from build123d import *

# Parameters (mm, degrees)
CORTE_EXTRUS_O1_DEPTH      = 14.238697312
CORTE_EXTRUS_O1_DEPTH_BACK = 14.238697312
ESBO_O2_W                  = 3.17038165
ESBO_O2_H                  = 1.5


with BuildPart() as part:
    # Esboço1 → Revolução1 (revolve)
    with BuildSketch(Plane.XY):
        with BuildLine():
            Line((0, 0), (0, 2.5))
            Line((0, 2.5), (8, 2.5))
            Line((8, 2.5), (8, 3.953675657))
            ThreePointArc((8, 3.953675657), (10.812174165, 2.798528059), (12, 0))
            Line((12, 0), (0, 0))
        make_face()
    revolve(axis=Axis((12, 0, 0), (-1, 0, 0)))

    # Esboço2 → Corte-extrusão1 (cut, two sides: drawn at the far end of the back side and taken through both)
    with BuildSketch(Plane.XY.offset(-CORTE_EXTRUS_O1_DEPTH_BACK)):
        with Locations((11.06193306, 0)):
            Rectangle(ESBO_O2_W, ESBO_O2_H)
    extrude(amount=CORTE_EXTRUS_O1_DEPTH + CORTE_EXTRUS_O1_DEPTH_BACK, mode=Mode.SUBTRACT)


solid = part.part
Work out the finished part from the listing and answer in its coordinate system (mm). A direction names the side the tool comes from. Coordinates: 2 decimals unless noted, no trailing zeros. Write each loop counter-clockwise with the first axis right and the second up, starting at its lowest first coordinate (ties: lowest second). Pieces come first, ordered by that corner, then holes. Notation, with made-up numbers: M 14,13 L 45,13 A37 cw 45,52 Z; hole C 7.25,25 d2. An arc over 180 degrees is marked long. Use one line per item in the form item = value. Start each with the question number.
1. Straight lines are drawn through the part: probe 1 along Y at (x, z) = (10, 2.25); probe 2 along X at (y, z) = (0.5, 1); probe 3 along Y at (x, z) = (10, 0.25). For each, find the intervals that lie inside material, in ascending order. Write a range as from..to.
2. The mould has two halves that part along Y. Classify faces 1 (the face through (4.06, -0.54, 2.44)), 2 (the face through (10, 0.75, 0)), 3 (the face through (0, 0, 0)), 4 (the face through (9.477, 0, 0)): released by +Y, released by -Y, zero draft, split by the parting line, or undercut.
3. A tool of negligible diameter and unlimited length cuts with its end or side. For faces 5 (the face through (8, 0, 3)), 6 (the face through (10, -0.75, 0)), from which of +Z, -Z, +X, -X, +Y, -Y can it reach the whole face along a straight path? Write none if from no direction.
4. The part is cut by section A-A (x = 4). Give the vertices of the cut face in (y, z).
5. Each of these flat-tipped pins is pushed along its axis until it touches: P1, Ø1, axis at y = 3, z = 0.5, coming from the +X side; P2, Ø1, axis at x = 9.5, y = -1.5, coming from the +Z side; P3, Ø0.7, axis at x = 10.5, z = -2, coming from the +Y side. Where does it stop, or does it pass through?
Evaluation:
q1.probe_1 = -2.57..-0.75, 0.75..2.57
q1.probe_2 = 0..9.48
q1.probe_3 = -3.41..-0.75, 0.75..3.41
q2.face_1 = split by the parting line
q2.face_2 = undercut
q2.face_3 = zero draft
q2.face_4 = undercut
q3.face_5 = -X
q3.face_6 = +Z, -Z, +X
q4.outline = C 0,0 d5
q5.P1 = 11.05
q5.P2 = 3.61
q5.P3 = 2.75
